from build123d import *

# Parameters (mm, degrees)
F0_W     = 25.4
F0_H     = 25.4
F2_DEPTH = 25.4
F3_DEPTH = 25.4


with BuildPart() as f2:
    # F0 (on Front) → F2 (new body)
    with BuildSketch(Plane.XZ):
        with Locations((12.7, 12.7)):
            Rectangle(F0_W, F0_H)
    extrude(amount=-F2_DEPTH)

    # F1 (on face) → F3 (cut)
    with BuildSketch(Plane.XZ):
        Polygon((0, 25.4), (0, 16.51), (5.08, 16.51), (2.274592, 19.087943), (8.275861, 19.728145), (3.726008, 21.337217), (16.39788, 22.182008), (14.994388, 23.235855), (22.614388, 23.235855), (19.311167, 21.337217), (23.86102, 19.728145), (19.311167, 18.119072), (23.86102, 16.51), (23.86102, 0), (25.4, 0), (25.4, 25.4), align=None)
        Polygon((9.083407, 15.24), (3.726008, 15.24), (6.652538, 12.90414), (9.083407, 12.90414), (12.361358, 12.90414), (14.740032, 12.90414), (16.960129, 11.318357), (19.311167, 12.90414), (19.311167, 15.24), align=None)
        Polygon((3.726008, 5.054513), (3.726008, 0), (19.311167, 0), (19.311167, 5.688827), (14.977898, 5.688827), (13.550695, 4.816646), (11.727044, 4.816646), (11.727044, 5.688827), (9.189791, 5.688827), (6.573249, 5.688827), (6.067413, 6.337257), (4.396382, 6.337257), align=None)
        Polygon((12.916381, 8.622526), (12.916381, 5.688827), (14.502165, 6.402429), (14.502165, 7.829634), align=None)
        Polygon((12.361358, 11.239068), (9.083407, 12.111248), (9.083407, 10.446176), (12.361358, 10.446176), align=None)
        Polygon((17.039418, 9.732574), (19.311167, 12.90414), (16.960129, 11.318357), (14.740032, 12.90414), align=None)
        Polygon((5.066755, 7.62), (4.396382, 6.337257), (6.067413, 6.337257), align=None)
    extrude(amount=-F3_DEPTH, mode=Mode.SUBTRACT)


solid = f2.part
Source: CAD feature listing. Evaluate the final solid. Frame: model axes, mm. A direction names the side the tool comes from. Coordinates: 2 decimals unless noted, no trailing zeros. Order: outer loops, then holes, each group sorted by start corner. A loop starts at its lowest first (then second) coordinate and runs counter-clockwise, first axis right, second up. Notation, with made-up numbers: M 83,15.25 L 133,15.25 A15 ccw 133,30.25 Z; hole C 88,72 d6. An arc over 180 degrees is marked long. Write each question's results on one line, items separated by ' | '. Start each with the question number.
1. Reachability of faces 1 (the face through (12, 13, 15.24)), 2 (the face through (11.727, 13, 5)), 3 (the face through (3.7, 12.52, 17.78)), 4 (the face through (21.554, 12.522, 17.326)) from +Z, -Z, +X, -X, +Y, -Y: full face, straight path, thin tool, end or side. Return the list, or none.
2. Section A-A, the plane z = 4.25. Return the cut outline in (x, y).
3. Section B-B, the plane x = 17.75. Return the cut outline in (y, z).
4. Draft query along X for faces 5 (the face through (5.2, 12.5, 19.4)), 6 (the face through (17, 13, 5.689)), 7 (the face through (12, 25.4, 12)). Return one class per face: +X half, -X half, draft (parallel to the pull), parting line (faces both ways), or undercut.
5. Material intervals for L1, parallel to X at y = 8, z = 2.5; L2, parallel to X at y = 8.5, z = 7.25; L3, parallel to Z at x = 11, y = 2.75, sorted ascending.
6. Section C-C, the plane x = 10.5. Return the cut outline in (y, z), then the cut area to 3 significant figures.
7. Section D-D, the plane y = 16. State how many separate pieces and enclosed holes the cut face has, then the cut area to 3 significant figures.
8. Pin query (flat end, axial travel): pin 1 (10 mm diameter, centred on x = 17, z = 10, fed in from -Y); pin 2 (3.5 mm diameter, centred on x = 11, y = 10.5, fed in from +Z); pin 3 (5 mm diameter, centred on x = 14, y = 13, fed in from -Z); pin 4 (2 mm diameter, centred on x = 18, y = 18, fed in from -Z). Return the tip coordinate at first contact, or that it passes through.
Solution:
1) face 1: +Y, -Y | face 2: -Z, +Y, -Y | face 3: -X, +Y, -Y | face 4: +X, +Y, -Y
2) outline: M 0,0 L 3.73,0 L 3.73,25.4 L 0,25.4 Z; M 19.31,0 L 23.86,0 L 23.86,25.4 L 19.31,25.4 Z
3) outline: M 0,5.69 L 25.4,5.69 L 25.4,10.72 L 0,10.72 Z; M 0,15.24 L 25.4,15.24 L 25.4,23.24 L 0,23.24 Z
4) face 5: -X half | face 6: undercut | face 7: draft
5) L1: 0 to 3.73, 19.31 to 23.86 | L2: 0 to 4.87, 5.36 to 12.92, 14.5 to 23.86 | L3: 5.69 to 10.45, 11.6 to 12.9, 15.24 to 21.82
6) outline: M 0,5.69 L 25.4,5.69 L 25.4,10.45 L 0,10.45 Z; M 0,11.73 L 25.4,11.73 L 25.4,12.9 L 0,12.9 Z; M 0,15.24 L 25.4,15.24 L 25.4,21.79 L 0,21.79 Z | area: 317 mm²
7) separate pieces: 1 | enclosed holes: 3 | area: 354 mm²
8) pin 1: y = 0 | pin 2: z = 21.94 | pin 3: z = 4.82 | pin 4: z = 5.69
